Model file for the job. Use its own axes, mm. A direction names the side the tool comes from. Give positions to 0.01 mm unless a question says otherwise; leave off trailing zeros. Write each loop counter-clockwise with the first axis right and the second up, starting at its lowest first coordinate (ties: lowest second). Pieces come first, ordered by that corner, then holes.
```python
from build123d import *

# Parameters (mm, degrees)
SKETCH1_R           = 4.445
BOSS_EXTRUDE1_DEPTH = 5.08
SKETCH1_8_R         = 4.445
BOSS_EXTRUDE2_DEPTH = 7.62


with BuildPart() as part:
    # Sketch1 → Boss-Extrude1 (new body)
    with BuildSketch(Plane.XY):
        with BuildLine():
            Line((-6.985, 0), (-6.985001912, 12.7))
            ThreePointArc((-6.985001912, 12.7), (-4.428413558, 18.101796467), (1.369871983, 19.549357814))
            Line((1.369871983, 19.549357814), (33.119871608, 13.199355939))
            ThreePointArc((33.119871608, 13.199355939), (38.735, 6.349999683), (33.119870986, -0.499356063))
            Line((33.119870986, -0.499356063), (1.369870986, -6.849355012))
            ThreePointArc((1.369870986, -6.849355012), (-4.428412185, -5.401794068), (-6.985, 0))
        make_face()
        with Locations((31.75, 6.35)):
            Circle(SKETCH1_R, mode=Mode.SUBTRACT)
        with BuildLine():
            Line((-4.445, 0), (-4.445, 12.7))
            ThreePointArc((-4.445, 12.7), (0, 17.145), (4.445, 12.7))
            Line((4.445, 12.7), (4.445, 0))
            ThreePointArc((4.445, 0), (0, -4.445), (-4.445, 0))
        make_face(mode=Mode.SUBTRACT)
    extrude(amount=BOSS_EXTRUDE1_DEPTH)

    # Sketch1_8 → Boss-Extrude2 (add)
    with BuildSketch(Plane.XY):
        with BuildLine():
            Line((4.445, 0), (4.445, 12.7))
            ThreePointArc((4.445, 12.7), (0, 17.145), (-4.445, 12.7))
            Line((-4.445, 12.7), (-4.445, 0))
            ThreePointArc((-4.445, 0), (0, -4.445), (4.445, 0))
        make_face()
        with Locations(Location((31.75, 6.35, 0), (0, 0, 180))):
            Circle(SKETCH1_8_R)
    extrude(amount=BOSS_EXTRUDE2_DEPTH)


solid = part.part
```
1. Slice it at D-D, the plane z = 4. Write the cut outline in (x, y) (3 decimals), and give its area (3 significant figures).
Calculated:
outline: (-6.985, 0) arc R6.985 ccw to (1.37, -6.849) - (33.12, -0.499) arc R6.985 ccw to (33.12, 13.199) - (1.37, 19.549) arc R6.985 ccw to (-6.985, 12.7) - close
area: 896 mm2
2. Which spindle directions (+Z, -Z, +X, -X, +Y, -Y) get a long thin tool onto all of the face, cutting with end or side? Do faces 1 (the flat face through (4.445, 6, 6)), 2 (the cylindrical face through (0.098, 17.144, 6.332)), 3 (the flat face through (-4.445, 6, 6)). Say none if no direction does.
Calculated:
face 1: +Z, +Y, -Y
face 2: +Z, +Y
face 3: +Z, -X, +Y, -Y
3. Pin check, flat tips, straight feed: P1, Ø3, axis at y = 4, z = 7, coming from the -X side (3 decimals); P2, Ø3, axis at y = 5, z = 6.5, coming from the +X side; P3, Ø1, axis at x = 10, y = 5, coming from the +Z side. Stop position of each tip, or through.
Calculated:
P1: stops at x = -4.445
P2: stops at x = 38.68
P3: stops at z = 5.08
4. Pull direction X, two halves, no side cores. Call faces 4 (the cylindrical face through (27.644, 8.052, 6.332)), 5 (the flat face through (16, 7, 5.08)), 6 (the cylindrical face through (38.734, 6.484, 2.504)), 7 (the cylindrical face through (-0.098, -4.444, 6.332)): +X half, -X half, draft (parallel to the pull), parting line (faces both ways), or undercut.
Calculated:
face 4: undercut
face 5: undercut
face 6: +X half
face 7: parting line
5. Probe probe 1 along Z at (x, y) = (22.5, -1); probe 2 along X at (y, z) = (8, 6.75) (3 decimals); probe 3 along X at (y, z) = (11.25, 3) (3 decimals). List the from-to ranges inside material, lowest first.
Calculated:
probe 1: z = 0 to 5.08
probe 2: x = -4.445 to 4.445, 27.623 to 35.877
probe 3: x = -6.985 to 36.728
6. Slice it at B-B, the plane y = 6.35. Write the cut outline in (x, z) (3 decimals), and give its area (3 significant figures).
Calculated:
outline: (-6.985, 0) - (38.735, 0) - (38.735, 5.08) - (36.195, 5.08) - (36.195, 7.62) - (27.305, 7.62) - (27.305, 5.08) - (4.445, 5.08) - (4.445, 7.62) - (-4.445, 7.62) - (-4.445, 5.08) - (-6.985, 5.08) - close
area: 277 mm2
7. Slice it at C-C, the plane x = 0. Write the cut outline in (y, z) (3 decimals).
Calculated:
outline: (-6.985, 0) - (19.685, 0) - (19.685, 5.08) - (17.145, 5.08) - (17.145, 7.62) - (-4.445, 7.62) - (-4.445, 5.08) - (-6.985, 5.08) - close
8. Slice it at A-A, the plane z = 7. Write the cut outline in (x, y) (3 decimals), and give its area (3 significant figures).
Calculated:
outline: (-4.445, 0) arc R4.445 ccw to (4.445, 0) - (4.445, 12.7) arc R4.445 ccw to (-4.445, 12.7) - close; circle Ø8.89 at (31.75, 6.35)
area: 237 mm2
